For this review, use the dimensioned drawing (mm, ordinates from the lowest corner) and the shaded views. Coordinates: 2 decimals unless noted, no trailing zeros. Loops run counter-clockwise (first coordinate to the right, second up) from the corner with the lowest first, then second, coordinate; pieces in that order, holes last. Notation, with made-up numbers: M -30,-0.5 L -7,-0.5 A23 cw -7,25.5 Z; hole C -26.75,69.5 d5. An arc over 180 degrees is marked long. Write item = value, one per line. Start each with the question number.
Q1. We need section C-C on y = 38.1. Give the boundary of the cut face in (x, z) (3 decimals).
Q2. We need section B-B on z = 0.95. Give the boundary of the cut face in (x, y) (3 decimals), and give its area (3 significant figures).
Q3. Clearance check with flat-ended pins moving along their axes: pin 1 Ø4 at (x, y) = (10, 12.7) entering from +Z; pin 2 Ø7 at (x, y) = (10, 80.8) entering from +Z. State where each tip first meets the part, or that it passes through.
Q4. Wall thickness on probe 1 along Y at (x, z) = (10, 2.95) (3 decimals); probe 2 along Y at (x, z) = (7.75, 0.95): over which ranges is each line inside the solid? List them lowest first.
Q5. We need section A-A on y = 60.8. Give the boundary of the cut face in (x, z), and give its area (3 significant figures).
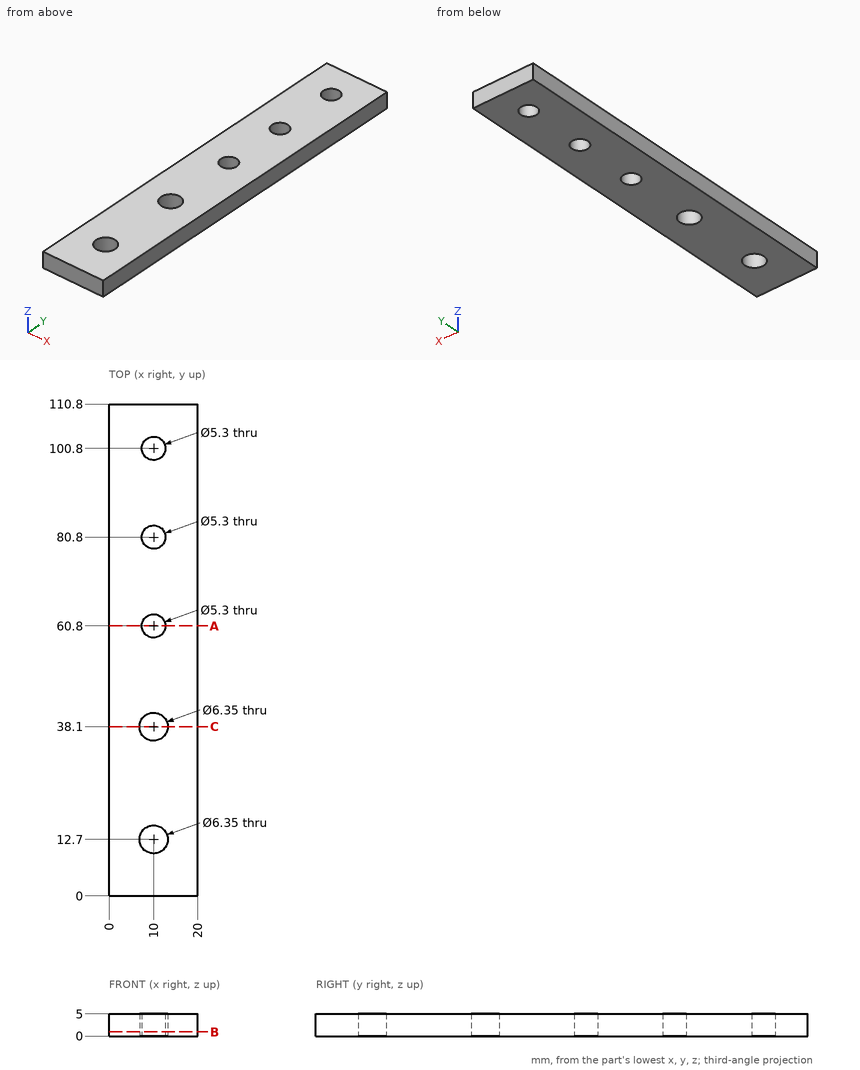
Returned:
q1.outline = M 0,0 L 6.825,0 L 6.825,5 L 0,5 Z; M 13.175,0 L 20,0 L 20,5 L 13.175,5 Z
q2.outline = M 0,0 L 20,0 L 20,110.8 L 0,110.8 Z; hole C 10,12.7 d6.35; hole C 10,38.1 d6.35; hole C 10,60.8 d5.3; hole C 10,80.8 d5.3; hole C 10,100.8 d5.3
q2.area = 2,090 mm^2
q3.pin_1 = through
q3.pin_2 = 5
q4.probe_1 = 0 to 9.525, 15.875 to 34.925, 41.275 to 58.15, 63.45 to 78.15, 83.45 to 98.15, 103.45 to 110.8
q4.probe_2 = 0 to 10.46, 14.94 to 35.86, 40.34 to 59.4, 62.2 to 79.4, 82.2 to 99.4, 102.2 to 110.8
q5.outline = M 0,0 L 7.35,0 L 7.35,5 L 0,5 Z; M 12.65,0 L 20,0 L 20,5 L 12.65,5 Z
q5.area = 73.5 mm^2
